The listing builds one solid part. Answer for the finished solid, in the listing's coordinates (mm). A direction names the side the tool comes from. Give positions to 0.01 mm unless a question says otherwise; leave off trailing zeros. Loops run counter-clockwise (first coordinate to the right, second up) from the corner with the lowest first, then second, coordinate; pieces in that order, holes last. Notation, with made-up numbers: (43, 68) - (66, 68) arc R20 cw to (66, 103) - close; hole circle Ø3 at (74.5, 74). An arc over 180 degrees is marked (long way). Write item = value, one per line. Start each with the question number.
1) Consider probe 1 along X at (y, z) = (-6, 1.3); probe 2 along Y at (x, z) = (2.25, 2.6); probe 3 along X at (y, z) = (6, 4.5). Determine where each line is inside the solid, lowest interval first.
2) The mould has two halves that part along Y. Classify faces 1 (the flat face through (-0.04, 7.01, 9.24)), 2 (the flat face through (3, 5.1, 8.3)), 3 (the cylindrical face through (-4, 0, 7)): +Y half, -Y half, draft (parallel to the pull), parting line (faces both ways), or undercut.
3) The part is cut by section C-C on y = -6. Write down the section's boundary in (x, z).
4) The part is cut by section D-D on z = 1.25. Write down the section's boundary in (x, y), plus the area to 3 significant figures.
5) The part is cut by section B-B on y = 6. Write down the section's boundary in (x, z).
6) The part is cut by section A-A on x = 2.25. Write down the section's boundary in (y, z), plus the area to 3 significant figures.
7) Which of the six approach directions +Z, -Z, +X, -X, +Y, -Y give full straight-line access (tool end or side, diameter ignored) to faces 4 (the cylindrical face through (2.536, -7.289, 4.677)), 5 (the flat face through (-3, 4.7, 7.8)), 6 (the flat face through (1, 4, 8))?
8) Flat-ended cylindrical pins translate along their axes: P1, Ø2, axis at x = 3.5, y = 0, coming from the +Z side; P2, Ø1.3, axis at y = 5.5, z = 8, coming from the -X side; P3, Ø1.5, axis at x = 0.5, z = 7, coming from the -Y side. Find the tip coordinate at first contact, or state that the pin passes through.
from build123d import *

# Parameters (mm, degrees)
F0_W      = 12
F0_H      = 15.5
F1_DEPTH  = 10
F3_DEPTH  = 4.5
F4_W      = 8.5
F4_H      = 3.5
F5_DEPTH  = 8
F6_R      = 3
F7_SIZE   = 1.5
F9_D      = 2
F9_DEPTH  = 3
F9_TIP    = 0.600860619
F12_W     = 5
F12_H     = 4.5
F13_DEPTH = 3
F14_R     = 3
F16_D     = 2
F18_D     = 1.5
F20_D     = 2.64
F20_DEPTH = 1.624
F20_TIP   = 0.7931360171
F21_SIZE  = 0.5
F23_D     = 2.4
F23_DEPTH = 6
F23_START = 0.2
F23_TIP   = 0.7210327428
F25_D     = 2.4
F25_DEPTH = 6
F25_START = 0.95
F25_TIP   = 0.7210327428


# Not quite as in the source:
# - a feature of the source that left no trace in its solid (it failed there, or was rolled back) is left out


with BuildPart() as f1:
    # F0 (on Top) → F1 (new body)
    with BuildSketch(Plane.XY):
        Rectangle(F0_W, F0_H)
    extrude(amount=F1_DEPTH)

    # F2 (on face) → F3 (cut)
    with BuildSketch(Plane.XY.offset(10)):
        Polygon((-2, -7.75), (6, -7.75), (6, 7.75), (3, 7.75), (3, 4), (-2, 4), align=None)
    extrude(amount=-F3_DEPTH, mode=Mode.SUBTRACT)

    # F4 (on face) → F5 (cut)
    with BuildSketch(Plane.YZ.offset(6)):
        with Locations((-0.25, 3.75)):
            Rectangle(F4_W, F4_H)
    extrude(amount=-F5_DEPTH, mode=Mode.SUBTRACT)

    # F6
    f6_edges = [f1.edges().sort_by_distance(p)[0] for p in [
        (2, 4, 2),
        (2, -4.5, 2),
    ]]
    fillet(f6_edges, radius=F6_R)

    # F7
    f7_edges = [f1.edges().sort_by_distance(p)[0] for p in [
        (-1.5, 7.75, 10),
        (0, -7.75, 0),
        (-4, -7.75, 10),
        (0, 7.75, 0),
    ]]
    chamfer(f7_edges, length=F7_SIZE)

    # F9
    with Locations(Plane(origin=(-6, 0, 0), x_dir=(0, -1, 0), z_dir=(-1, 0, 0))):
        with Locations((0, 6)):
            Hole(F9_D / 2, depth=F9_DEPTH)
            with Locations((0, 0, -(F9_DEPTH + F9_TIP / 2))):  # 118° drill point
                Cone(0, F9_D / 2, F9_TIP, mode=Mode.SUBTRACT)

    # F12 (on face) → F13 (cut)
    with BuildSketch(Plane(origin=(-6, 0, 0), x_dir=(0, -1, 0), z_dir=(-1, 0, 0))):
        with Locations((-5.25, 7.75)):
            Rectangle(F12_W, F12_H)
    extrude(amount=-F13_DEPTH, mode=Mode.SUBTRACT)

    # F14
    f14_edges = [f1.edges().sort_by_distance(p)[0] for p in [
        (-4.5, 2.75, 5.5),
    ]]
    fillet(f14_edges, radius=F14_R)

    # F16 (through all)
    with Locations(Plane(origin=(-3, 0, 0), x_dir=(0, -1, 0), z_dir=(-1, 0, 0))):
        with Locations((-6, 7.5)):
            Hole(F16_D / 2)

    # F18 (through all)
    with Locations(Plane.XY.offset(5.5)):
        with Locations((2.25, -6)):
            Hole(F18_D / 2)

    # F20
    with Locations(Plane.XY.offset(5.5)):
        with Locations((2.25, -6)):
            Hole(F20_D / 2, depth=F20_DEPTH)
            with Locations((0, 0, -(F20_DEPTH + F20_TIP / 2))):  # 118° drill point
                Cone(0, F20_D / 2, F20_TIP, mode=Mode.SUBTRACT)

    # F21
    f21_edges = [f1.edges().sort_by_distance(p)[0] for p in [
        (-6, -1.75, 10),
        (6, -6.125, 5.5),
        (6, 5.875, 5.5),
        (6, 7.75, 3.5),
        (6, 0, 0),
        (-6, 0, 0),
        (-6, -7.75, 5),
        (-6, 7.75, 3.5),
        (6, -7.75, 3.5),
    ]]
    chamfer(f21_edges, length=F21_SIZE)

    # F23
    # its depths count from where the whole tool has entered the part; down to there all is cleared
    with Locations(Plane(origin=(0, 0, 0), x_dir=(1, 0, 0), z_dir=(0, 0, -1)).offset(-F23_START)):
        with Locations((-4.5, 0)):
            Hole(F23_D / 2, depth=F23_DEPTH)
            with Locations((0, 0, -(F23_DEPTH + F23_TIP / 2))):  # 118° drill point
                Cone(0, F23_D / 2, F23_TIP, mode=Mode.SUBTRACT)

    # F25
    # its depths count from where the whole tool has entered the part; down to there all is cleared
    with Locations(Plane(origin=(0, 0, 0), x_dir=(1, 0, 0), z_dir=(0, 0, -1)).offset(-F25_START)):
        with Locations((0, -6)):
            Hole(F25_D / 2, depth=F25_DEPTH)
            with Locations((0, 0, -(F25_DEPTH + F25_TIP / 2))):  # 118° drill point
                Cone(0, F25_D / 2, F25_TIP, mode=Mode.SUBTRACT)


solid = f1.part
Answer below:
q1.probe_1 = -6 to 1.5, 3 to 6
q1.probe_2 = -7.75 to -6.75, -5.25 to -3.3, 2.8 to 7.75
q1.probe_3 = -6 to -1.2, 1.2 to 6
q2.face_1 = +Y half
q2.face_2 = draft
q2.face_3 = undercut
q3.outline = (-6, 0.5) - (-5.5, 0) - (1.5, 0) - (1.5, 3.53) - (0.93, 3.88) - (0.93, 5.5) - (-2, 5.5) - (-2, 10) - (-5.5, 10) - (-6, 9.5) - close; (3, 0) - (5.5, 0) - (6, 0.5) - (6, 5) - (5.5, 5.5) - (3.57, 5.5) - (3.57, 3.88) - (3, 3.53) - close
q4.outline = (-6, -7.25) - (-5.75, -7.5) - (5.75, -7.5) - (6, -7.25) - (6, 7.25) - (5.75, 7.5) - (-5.75, 7.5) - (-6, 7.25) - close; hole circle Ø2.4 at (-4.5, 0); hole circle Ø2.4 at (0, 6); hole circle Ø1.5 at (2.25, -6)
q4.area = 169 mm2
q5.outline = (-6, 0.5) - (-5.5, 0) - (-1.2, 0) - (-1.2, 6.5) - (-3, 6.5) - (-3, 5.5) - (-6, 5.5) - close; (-3, 8.5) - (3, 8.5) - (3, 10) - (-3, 10) - close; (1.2, 0) - (5.5, 0) - (6, 0.5) - (6, 5) - (5.5, 5.5) - (3, 5.5) - (3, 6.5) - (1.2, 6.5) - close
q6.outline = (-7.75, 1.5) - (-6.75, 0.5) - (-6.75, 3.53) - (-7.32, 3.88) - (-7.32, 5.5) - (-7.75, 5.5) - close; (-5.25, 0) - (6.25, 0) - (7.75, 1.5) - (7.75, 8.5) - (6.25, 10) - (4, 10) - (4, 5) arc R3 cw to (1, 2) - (-1.5, 2) arc R3 cw to (-4.5, 5) - (-4.5, 5.5) - (-4.68, 5.5) - (-4.68, 3.88) - (-5.25, 3.53) - close; hole circle Ø2 at (6, 7.5)
q6.area = 59.5 mm2
q7.face_4 = +Z
q7.face_5 = +Z, -X, +Y
q7.face_6 = +Z, +X
q8.P1 = 2
q8.P2 = -3
q8.P3 = 4
